Autodesk Inventor part; units mm, degrees
ref_plane "YZ Plane" through (0, 0, 0) normal (1, 0, 0) x (0, 1, 0)
ref_plane "XZ Plane" through (0, 0, 0) normal (0, 1, 0) x (-1, 0, 0)
ref_plane "XY Plane" through (0, 0, 0) normal (0, 0, 1) x (1, 0, 0)
sketch "Skizze9" plane through (0, 0, 0) normal (0, 1, 0) x (-1, 0, 0)
  line L0 (4.275, 15.405) -> (-4.275, 15.405)
  line L1 (-6.275, 13.405) -> (-6.275, -13.405)
  line L2 (-4.275, -15.405) -> (4.275, -15.405)
  line L3 (6.275, -13.405) -> (6.275, 13.405)
  line L4 (0, 0) -> (0, -15.405) construction
  line L5 (0, 0) -> (6.275, 0) construction
  arc A0 (6.275, 13.405) -> (4.275, 15.405) centre (4.275, 13.405) ccw
  arc A1 (-6.275, -13.405) -> (-4.275, -15.405) centre (-4.275, -13.405) ccw
  arc A2 (4.275, -15.405) -> (6.275, -13.405) centre (4.275, -13.405) ccw
  arc A3 (-4.275, 15.405) -> (-6.275, 13.405) centre (-4.275, 13.405) ccw
  point P0 (6.275, 15.405)
  point P1 (-6.275, -15.405)
  point P2 (-6.275, 15.405)
  point P3 (6.275, -15.405)
  dimension "d41" = 30.81
  dimension "d42" = 12.55
  dimension "d61" = 2
extrude "Extrusion6" add sketch "Skizze9" along normal blind 1
sketch "Skizze10" plane through (0, 1, 0) normal (0, 1, 0) x (1, 0, 0)
  line L0 (-4.275, -15.405) -> (4.275, -15.405)
  line L1 (6.275, -13.405) -> (6.275, 13.405)
  line L2 (4.275, 15.405) -> (-4.275, 15.405)
  line L3 (-6.275, 13.405) -> (-6.275, -13.405)
  line L4 (4.6, -6.0831) -> (4.6, 6.0831)
  line L5 (2.9473, 8.0527) -> (-2.2527, 8.9696)
  line L6 (-4.6, 7) -> (-4.6, -7)
  line L7 (-2.2527, -8.9696) -> (2.9473, -8.0527)
  line L8 (0, 0) -> (-4.6, 0) construction
  line L9 (0, 0) -> (4.6, 0) construction
  line L10 (-4.6, -9.3835) -> (6.275, -9.3835) construction
  line L11 (-4.6, 9.3835) -> (6.275, 9.3835) construction
  arc A0 (-4.6, -7) -> (-2.2527, -8.9696) centre (-2.6, -7) ccw
  arc A1 (-2.2527, 8.9696) -> (-4.6, 7) centre (-2.6, 7) ccw
  arc A2 (2.9473, -8.0527) -> (4.6, -6.0831) centre (2.6, -6.0831) ccw
  arc A3 (4.6, 6.0831) -> (2.9473, 8.0527) centre (2.6, 6.0831) ccw
  arc A4 (4.275, -15.405) -> (6.275, -13.405) centre (4.275, -13.405) ccw
  arc A5 (6.275, 13.405) -> (4.275, 15.405) centre (4.275, 13.405) ccw
  arc A6 (-4.275, 15.405) -> (-6.275, 13.405) centre (-4.275, 13.405) ccw
  arc A7 (-6.275, -13.405) -> (-4.275, -15.405) centre (-4.275, -13.405) ccw
  dimension "d45" = 10
  dimension "d46" = 4.6
  dimension "d47" = 4.6
  dimension "d49" = 2
  dimension "d67" = 14
  dimension "d68" = 18
extrude "Extrusion7" add sketch "Skizze10" along normal blind 6.1 contours A2 L7 A0 L6 A1 L5 A3 L4
sketch "Skizze11" plane through (0, 1, 0) normal (0, 1, 0) x (1, 0, 0)
  arc A0 (-2.2527, 8.9696) -> (-4.6, 7) centre (-2.6, 7) ccw
  line L0 (-2.2527, 8.9696) -> (2.9473, 8.0527)
  arc A1 (4.6, 6.0831) -> (2.9473, 8.0527) centre (2.6, 6.0831) ccw
  line L1 (4.6, 6.0831) -> (4.6, -6.0831)
  arc A2 (2.9473, -8.0527) -> (4.6, -6.0831) centre (2.6, -6.0831) ccw
  line L2 (2.9473, -8.0527) -> (-2.2527, -8.9696)
  arc A3 (-4.6, -7) -> (-2.2527, -8.9696) centre (-2.6, -7) ccw
  line L3 (-4.6, -7) -> (-4.6, 7)
  line L4 (-4.275, -15.405) -> (4.275, -15.405)
  line L5 (6.275, -13.405) -> (6.275, 13.405)
  line L6 (4.275, 15.405) -> (-4.275, 15.405)
  line L7 (-6.275, 13.405) -> (-6.275, -13.405)
  line L8 (0, 0) -> (0, 12.5) construction
  line L9 (0, 0) -> (0, -12.5) construction
  arc A4 (4.275, -15.405) -> (6.275, -13.405) centre (4.275, -13.405) ccw
  arc A5 (6.275, 13.405) -> (4.275, 15.405) centre (4.275, 13.405) ccw
  arc A6 (-4.275, 15.405) -> (-6.275, 13.405) centre (-4.275, 13.405) ccw
  arc A7 (-6.275, -13.405) -> (-4.275, -15.405) centre (-4.275, -13.405) ccw
  dimension "d52" = 12.5
  dimension "d53" = 12.5
hole "Bohrung3" at (0, 1, 12.5) at (0, 1, -12.5) direction (0, -1, 0) diameter 3.3 end through all
sketch "Skizze12" plane through (0, 0, 0) normal (0, -1, 0) x (1, 0, 0)
  circle A0 centre (0, 12.5) radius 1.65
  circle A1 centre (0, -12.5) radius 1.65
  line L0 (-4.275, 15.405) -> (4.275, 15.405)
  arc A2 (-4.275, 15.405) -> (-6.275, 13.405) centre (-4.275, 13.405) ccw
  line L1 (-6.275, -13.405) -> (-6.275, 13.405)
  arc A3 (-6.275, -13.405) -> (-4.275, -15.405) centre (-4.275, -13.405) ccw
  line L2 (4.275, -15.405) -> (-4.275, -15.405)
  arc A4 (4.275, -15.405) -> (6.275, -13.405) centre (4.275, -13.405) ccw
  line L3 (6.275, 13.405) -> (6.275, -13.405)
  arc A5 (6.275, 13.405) -> (4.275, 15.405) centre (4.275, 13.405) ccw
  line L4 (-5.55, -8.46) -> (5.55, -8.46)
  line L5 (5.55, -8.46) -> (5.55, 8.46)
  line L6 (5.55, 8.46) -> (-5.55, 8.46)
  line L7 (-5.55, 8.46) -> (-5.55, -8.46)
  line L8 (0, 0) -> (0, 8.46) construction
  line L9 (0, 0) -> (-5.55, 0) construction
  dimension "d62" = 11.1
  dimension "d63" = 16.92
extrude "Extrusion8" add sketch "Skizze12" along normal blind 12.5 contours L7 L6 L5 L4
properties part number "anschluss_daten_2"
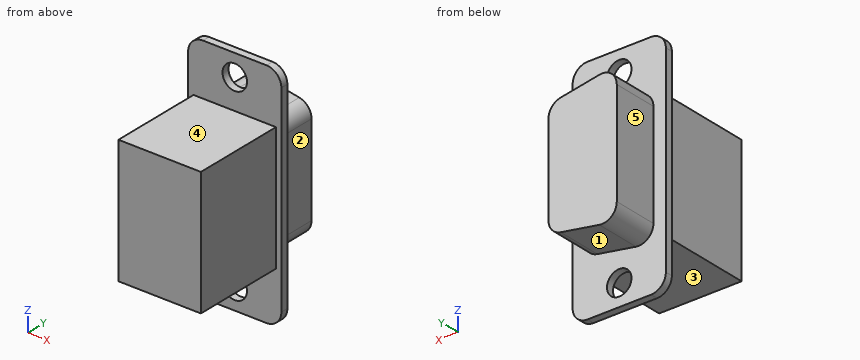
Geometry check sheet. Reference: the model listing, model coordinates, mm. Face numbers are marked on the shaded views. A direction names the side the tool comes from. Coordinates: 2 decimals unless noted, no trailing zeros. Loops run counter-clockwise (first coordinate to the right, second up) from the corner with the lowest first, then second, coordinate; pieces in that order, holes last. Notation, with made-up numbers: (58, 4) - (72, 4) arc R23 ccw to (72, 32) - close; hole circle Ø4 at (59.25, 87.5). An arc over 180 degrees is marked (long way). Use one line per item in the form item = value. Start each with the question number.
Item 1: Section check B-B, the plane z = -4. Enter the section's corners in (x, y) (3 decimals).
Item 2: Section check C-C, the plane x = 0. Enter the section's corners in (y, z) (3 decimals).
Item 3: Section check A-A, the plane z = 12.5. Enter the section's corners in (x, y) (3 decimals), and give its area (3 significant figures).
Item 4: Section check D-D, the plane y = -1.75. Enter the section's corners in (x, z), and give its area (3 significant figures).
Item 5: Tool access check on the marked faces 1, 2, 3, 4 and 5. Record the directions out of +Z, -Z, +X, -X, +Y, -Y that give a thin tool (end or side, any length) a straight path to the whole face; none if there is none.
Item 6: Thickness scan on probe 1 along Z at (x, y) = (0, 0.4) (3 decimals); probe 2 along X at (y, z) = (0.5, 12.5) (3 decimals); probe 3 along Z at (x, y) = (3, -9). Record the ranges inside material, lowest first.
Item 7: Gauge pin test, flat ends, axial feed: pin 1 (4 mm diameter, centred on x = -1, y = 3.5, fed in from -Z); pin 2 (6.5 mm diameter, centred on y = 4, z = 0, fed in from +X) (3 decimals); pin 3 (1.5 mm diameter, centred on x = 4.5, z = 10.5, fed in from -Y); pin 4 (4 mm diameter, centred on y = -5, z = 3, fed in from -X). Record the tip position at first contact, or that the pin passes through.
Computed:
q1.outline = (-6.275, 0) - (-5.55, 0) - (-5.55, -12.5) - (5.55, -12.5) - (5.55, 0) - (6.275, 0) - (6.275, 1) - (4.6, 1) - (4.6, 7.1) - (-4.6, 7.1) - (-4.6, 1) - (-6.275, 1) - close
q2.outline = (-12.5, -8.46) - (0, -8.46) - (0, -10.85) - (1, -10.85) - (1, -8.572) - (7.1, -8.572) - (7.1, 8.572) - (1, 8.572) - (1, 10.85) - (0, 10.85) - (0, 8.46) - (-12.5, 8.46) - close; (0, -15.405) - (1, -15.405) - (1, -14.15) - (0, -14.15) - close; (0, 14.15) - (1, 14.15) - (1, 15.405) - (0, 15.405) - close
q3.outline = (-6.275, 0) - (-1.65, 0) - (-1.65, 1) - (-6.275, 1) - close; (1.65, 0) - (6.275, 0) - (6.275, 1) - (1.65, 1) - close
q3.area = 9.25 mm2
q4.outline = (-5.55, -8.46) - (5.55, -8.46) - (5.55, 8.46) - (-5.55, 8.46) - close
q4.area = 188 mm2
q5.face_1 = -Z, +X, +Y
q5.face_2 = +Z, -Z, +X, +Y
q5.face_3 = -Z, +X, -X, -Y
q5.face_4 = +Z, +X, -X, -Y
q5.face_5 = +Z, -Z, -X, +Y
q6.probe_1 = -15.405 to -14.15, -10.85 to 10.85, 14.15 to 15.405
q6.probe_2 = -6.275 to -1.65, 1.65 to 6.275
q6.probe_3 = -8.46 to 8.46
q7.pin_1 = -9
q7.pin_2 = 6.275
q7.pin_3 = 0
q7.pin_4 = -5.55
